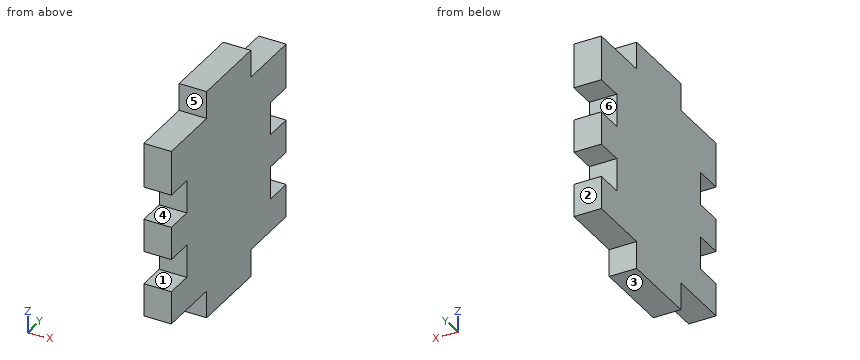
Autodesk Inventor part; units mm, degrees
ref_plane "YZ Plane" through (0, 0, 0) normal (1, 0, 0) x (0, 1, 0)
ref_plane "XZ Plane" through (0, 0, 0) normal (0, 1, 0) x (-1, 0, 0)
ref_plane "XY Plane" through (0, 0, 0) normal (0, 0, 1) x (1, 0, 0)
sketch "Sketch1" plane through (0, 0, 0) normal (1, 0, 0) x (0, 1, 0)
  line L0 (13, -14.75) -> (-13, -14.75)
  line L1 (-13, -14.75) -> (-13, 14.75) construction
  line L2 (-13, 14.75) -> (13, 14.75)
  line L3 (13, 14.75) -> (13, -14.75)
  line L4 (5, -14.75) -> (-5, -14.75)
  line L5 (-5, -14.75) -> (-5, -11.25)
  line L6 (-5, -11.25) -> (5, -11.25)
  line L7 (5, -11.25) -> (5, -14.75)
  line L8 (-5, -11.25) -> (-13, -11.25)
  line L9 (-13, -11.25) -> (-13, -7.05)
  line L10 (-13, -7.05) -> (-9.5, -7.05)
  line L11 (-9.5, -7.05) -> (-9.5, -2.85)
  line L12 (-9.5, -2.85) -> (-13, -2.85)
  line L13 (-13, -2.85) -> (-13, 1.35)
  line L14 (-13, 1.35) -> (-9.5, 1.35)
  line L15 (-9.5, 1.35) -> (-9.5, 5.55)
  line L16 (-9.5, 5.55) -> (-13, 5.55)
  line L17 (5, 14.75) -> (-5, 14.75)
  line L18 (-5, 14.75) -> (-5, 11.25)
  line L19 (-5, 11.25) -> (5, 11.25)
  line L20 (5, 11.25) -> (5, 14.75)
  line L21 (-5, 11.25) -> (-13, 11.25)
  line L22 (0, 0) -> (0, -1.9359)
  line L23 (5, -11.25) -> (13, -11.25)
  line L24 (13, -7.05) -> (9.5, -7.05)
  line L25 (9.5, -7.05) -> (9.5, -2.85)
  line L26 (9.5, -2.85) -> (13, -2.85)
  line L27 (13, 1.35) -> (9.5, 1.35)
  line L28 (9.5, 1.35) -> (9.5, 5.55)
  line L29 (9.5, 5.55) -> (13, 5.55)
  line L30 (5, 11.25) -> (13, 11.25)
  line L31 (-13, 11.25) -> (-13, 5.55)
  line L32 (-13, 1.35) -> (-13, -2.85)
  line L33 (-13, -7.05) -> (-13, -11.25)
  point P0 (0, -14.75)
  point P1 (-13, 0)
  point P2 (0, -11.25)
  point P3 (-5, -14.75)
  dimension "d0" = 26
  dimension "d1" = 29.5
  dimension "d2" = 10
  dimension "d3" = 3.5
  dimension "d4" = 4.2
  dimension "d5" = 3.5
  dimension "d6" = 4.2
  dimension "d7" = 4.2
  dimension "d8" = 4.2
  dimension "d9" = 3.5
extrude "Extrusion1" add sketch "Sketch1" along normal mid plane 3.5 contours L0 L5 L6 L7 | L23 L6 L8 L9 L10 L11 L12 L13 L14 L15 L16 L31 L21 L19 L30 L3 L29 L28 L27 L26 L25 L24 | L19 L18 L2 L20
sketch "Sketch2" plane through (1.75, 0, 0) normal (1, 0, 0) x (0, 0, -1)
  point P0 (0, 0)
properties part number "Stran Stran"
Geometry check sheet. Reference: the model listing, model coordinates, mm. Face numbers are marked on the shaded views. A direction names the side the tool comes from. Coordinates: 2 decimals unless noted, no trailing zeros. Order: outer loops, then holes, each group sorted by start corner. A loop starts at its lowest first (then second) coordinate and runs counter-clockwise, first axis right, second up. Notation, with made-up numbers: M -32.5,-35.75 L -4.5,-35.75 A21 ccw -4.5,-30.75 Z; hole C 43.25,29.25 d9. An arc over 180 degrees is marked long. Use CSV: the item, a comma, the result in double quotes.
Item 1: Thickness scan on line 1 along Z through (x, y) = (1, 10.75); line 2 along Y through (x, z) = (1.25, -12.25); line 3 along Y through (x, z) = (-1.45, -3.5). Record the ranges inside material, lowest first.
Returned:
line 1,"z = -11.25 to -7.05, -2.85 to 1.35, 5.55 to 11.25"
line 2,"y = -5 to 5"
line 3,"y = -9.5 to 9.5"
Item 2: Cross-section at D-D on z = 2.25. Record the cut outline in (x, y), then the cut area to 3 significant figures.
Returned:
outline,"M -1.75,-9.5 L 1.75,-9.5 L 1.75,9.5 L -1.75,9.5 Z"
area,"66.5 mm2"
Item 3: Mould release check, pull along Z, two halves, no side actions. Record for the marked faces 1, 2 and 3: pulls with the +Z half, pulls with the -Z half, needs draft (parallel to the pull), parting line crosses it, or undercut.
Returned:
face 1,"undercut"
face 2,"needs draft"
face 3,"pulls with the -Z half"
Item 4: Cross-section at B-B on x = -0.55. Record the cut outline in (y, z).
Returned:
outline,"M -13,-11.25 L -5,-11.25 L -5,-14.75 L 5,-14.75 L 5,-11.25 L 13,-11.25 L 13,-7.05 L 9.5,-7.05 L 9.5,-2.85 L 13,-2.85 L 13,1.35 L 9.5,1.35 L 9.5,5.55 L 13,5.55 L 13,11.25 L 5,11.25 L 5,14.75 L -5,14.75 L -5,11.25 L -13,11.25 L -13,5.55 L -9.5,5.55 L -9.5,1.35 L -13,1.35 L -13,-2.85 L -9.5,-2.85 L -9.5,-7.05 L -13,-7.05 Z"
Item 5: Cross-section at C-C on y = 7.5. Record the cut outline in (x, z).
Returned:
outline,"M -1.75,-11.25 L 1.75,-11.25 L 1.75,11.25 L -1.75,11.25 Z"
Item 6: Tool access check on the marked faces 4, 5 and 6. Record the directions out of +Z, -Z, +X, -X, +Y, -Y that give a thin tool (end or side, any length) a straight path to the whole face; none if there is none.
Returned:
face 4,"+X, -X, -Y"
face 5,"+Z, +X, -X, -Y"
face 6,"+X, -X, +Y"
Item 7: Cross-section at A-A on y = 11. Record the cut outline in (x, z), then the cut area to 4 significant figures.
Returned:
outline,"M -1.75,-11.25 L 1.75,-11.25 L 1.75,-7.05 L -1.75,-7.05 Z; M -1.75,-2.85 L 1.75,-2.85 L 1.75,1.35 L -1.75,1.35 Z; M -1.75,5.55 L 1.75,5.55 L 1.75,11.25 L -1.75,11.25 Z"
area,"49.35 mm2"
Item 8: Gauge pin test, flat ends, axial feed: pin 1 Ø1 at (x, y) = (-0.5, 10.5) entering from +Z; pin 2 Ø1 at (x, z) = (0.5, 2.5) entering from -Y. Record the tip position at first contact, or that the pin passes through.
Returned:
pin 1,"stops at z = 11.25"
pin 2,"stops at y = -9.5"
